```python
from build123d import *

# Parameters (mm, degrees)
PROFILEBOSS_EXTRUDE1_DEPTH      = 31.75
RIGHTPROFILEBOSS_EXTRUDE2_DEPTH = 68.25
SKETCH6_W                       = 5
SKETCH6_H                       = 62.32526864
TOPPROFILEBOSS_EXTRUDE5_DEPTH   = 65
SKETCH7_R                       = 2.25
HDMI_HOLESCUT_EXTRUDE1_DEPTH    = 130.147862652
SKETCH8_R                       = 1.5875
MOUNTHOLESCUT_EXTRUDE2_DEPTH    = 170.880700314
SKETCH9_R                       = 2.6
HDMIBORECUT_EXTRUDE3_DEPTH      = 1


with BuildPart() as part:
    # Sketch1 → ProfileBoss-Extrude1 (new body)
    with BuildSketch(Plane(origin=(0, 0, 0), x_dir=(1, 0, 0), z_dir=(0, 1, 0))):
        Polygon((0, 0), (0, 31.75), (65.532163543, 77.636114908), (65.532163543, 82.452293716), (56.390027919, 91.594429339), (59.925561825, 95.129963245), (70.532163543, 84.523361528), (70.532163543, 75.033279655), (5, 29.147164747), (5, 0), align=None)
    extrude(amount=PROFILEBOSS_EXTRUDE1_DEPTH)

    # Sketch2 → RightProfileBoss-Extrude2 (add)
    with BuildSketch(Plane.XZ):
        Polygon((59.925561825, -95.129963245), (70.532163543, -84.523361528), (70.532163543, -77.452293716), (65.532163543, -82.452293716), (56.390027919, -91.594429339), align=None)
    extrude(amount=RIGHTPROFILEBOSS_EXTRUDE2_DEPTH)

    # Sketch6 → TopProfileBoss-Extrude5 (add)
    with BuildSketch(Plane(origin=(-17.60220071, 0, -17.60220071), x_dir=(-0.7071067811865449, 0, 0.7071067811865502), z_dir=(-0.7071067811865502, 0, -0.7071067811865449))):
        with Locations((-107.140813238, -37.08736568)):
            Rectangle(SKETCH6_W, SKETCH6_H)
    extrude(amount=TOPPROFILEBOSS_EXTRUDE5_DEPTH)

    # Sketch7 → HDMI HolesCut-Extrude1 (cut, through all)
    with BuildSketch(Plane(origin=(77.527762535, 0, -77.527762535), x_dir=(-0.7071067811865493, 0, -0.7071067811865457), z_dir=(0.7071067811865457, 0, -0.7071067811865493))):
        with Locations((82.893270972, -11.25)):
            Circle(SKETCH7_R)
        with Locations((57.893270972, -11.25)):
            Circle(SKETCH7_R)
        with Locations((82.893270972, -61.25)):
            Circle(SKETCH7_R)
        with Locations((57.893270972, -61.25)):
            Circle(SKETCH7_R)
    extrude(amount=-HDMI_HOLESCUT_EXTRUDE1_DEPTH, mode=Mode.SUBTRACT)

    # Sketch8 → MountHolesCut-Extrude2 (cut, through all)
    with BuildSketch(Plane(origin=(5, 0, 0), x_dir=(0, 0, -1), z_dir=(1, 0, 0))):
        with Locations((7.9375, 23.8125)):
            Circle(SKETCH8_R)
        with Locations((21.209664747, 17.4625)):
            Circle(SKETCH8_R)
        with Locations((7.9375, 11.1125)):
            Circle(SKETCH8_R)
    extrude(amount=-MOUNTHOLESCUT_EXTRUDE2_DEPTH, mode=Mode.SUBTRACT)

    # Sketch9 → HDMIBoreCut-Extrude3 (cut)
    with BuildSketch(Plane(origin=(77.527762535, 0, -77.527762535), x_dir=(-0.7071067811865493, 0, -0.7071067811865457), z_dir=(0.7071067811865457, 0, -0.7071067811865493))):
        with Locations((57.893270972, -11.25)):
            Circle(SKETCH9_R)
        with Locations((82.893270972, -11.25)):
            Circle(SKETCH9_R)
        with Locations((82.893270972, -61.25)):
            Circle(SKETCH9_R)
        with Locations((57.893270972, -61.25)):
            Circle(SKETCH9_R)
    extrude(amount=-HDMIBORECUT_EXTRUDE3_DEPTH, mode=Mode.SUBTRACT)


solid = part.part
```
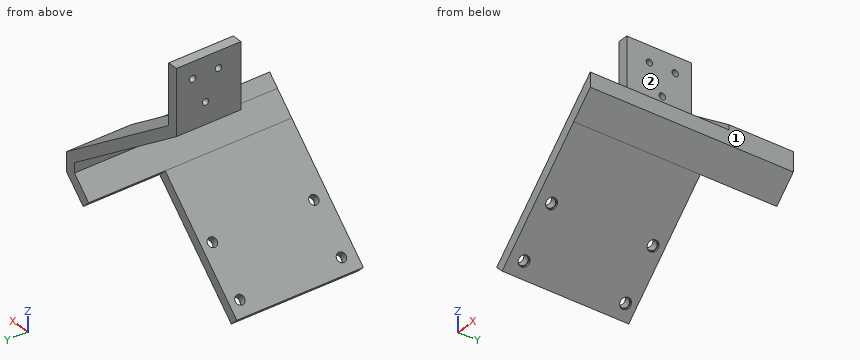
Could you check a few things on this model? Use its own coordinates, in mm. Face numbers are marked on the shaded views. A direction names the side the tool comes from. Give positions to 0.01 mm unless a question says otherwise; leave off trailing zeros. Loops run counter-clockwise (first coordinate to the right, second up) from the corner with the lowest first, then second, coordinate; pieces in that order, holes last. Notation, with made-up numbers: (-20, 66.25) - (2, 66.25) arc R28 cw to (2, 105.25) - close; hole circle Ø8 at (60, 20.25). An arc over 180 degrees is marked (long way). Use one line per item in the form item = value.
1. I want a section at D-D (x = 7.5). Please give me the cut outline in (y, z).
Response values:
outline = (0, -37) - (31.75, -37) - (31.75, -30.9) - (0, -30.9) - close
2. I want a section at B-B (x = 51). Please give me the cut outline in (y, z), and give its area (3 significant figures).
Response values:
outline = (-68.25, -104.06) - (-5.92, -104.06) - (-5.92, -96.98) - (-68.25, -96.98) - close; (0, -67.46) - (31.75, -67.46) - (31.75, -61.36) - (0, -61.36) - close
area = 635 mm²
3. On a 3-axis mill with a long thin cutter (end or side, diameter ignored), from which of +Z, -Z, +X, -X, +Y, -Y can I reach the whole of each face in a straight line? I mean the marked faces 1 and 2. Say none if no direction works.
Response values:
face_1 = +Z, -Z, +X, +Y, -Y
face_2 = +Z, +X, +Y, -Y
4. I want a section at A-A (y = -40). Please give me the cut outline in (x, z).
Response values:
outline = (10.43, -137.56) - (13.96, -141.09) - (70.53, -84.52) - (70.53, -77.45) - close
5. I'm going to push flat-ended pins straight in: pin 1 Ø12 at (x, y) = (46, -25.5) entering from -Z; pin 2 Ø2.5 at (y, z) = (9, -79) entering from -X; pin 3 Ø3 at (y, z) = (23.81, -7.94) entering from +X; pin 4 Ø24.5 at (x, z) = (47, -114) entering from +Y. Where does each tip first touch, or does it pass through?
Response values:
pin_1 = -115.06
pin_2 = 65.53
pin_3 = through
pin_4 = -5.92
6. I need wall thicknesses on probe 1 along X at (y, z) = (27.5, -25); probe 2 along Z at (x, y) = (64, -35); probe 3 along X at (y, z) = (-53.5, -93). Which ranges of each line are inside material? Lowest first, please.
Response values:
probe_1 = 0 to 5
probe_2 = -91.06 to -83.98
probe_3 = 54.98 to 62.06
7. I want a section at C-C (z = -42.5). Please give me the cut outline in (x, y), and give its area (3 significant figures).
Response values:
outline = (15.35, 0) - (24.07, 0) - (24.07, 31.75) - (15.35, 31.75) - close
area = 277 mm²
